from build123d import *

# Parameters (mm, degrees)
F2_R     = 0.4490128061
F3_DEPTH = 1.5875
F4_R     = 0.508


# Not quite as in the source:
# - a length typed as a fraction of an inch, garbled in the dataset ("3 / 203.2 mm" for 3/8 in), is restored


with BuildPart() as f3:
    # F2 (on Top) → F3 (new body)
    with BuildSketch(Plane.XY):
        Polygon((9.1678125, 1.27), (9.1678125, 4.0878125), (16.2321875, 4.0878125), (16.2321875, 1.27), (25.2002304245, 1.27), (25.2002304245, 17.78), (0, 17.78), (0, 1.27), align=None)
        with Locations((10.16, 7.62)):
            Circle(F2_R, mode=Mode.SUBTRACT)
        with Locations((12.7, 7.62)):
            Circle(F2_R, mode=Mode.SUBTRACT)
        with Locations((15.24, 7.62)):
            Circle(F2_R, mode=Mode.SUBTRACT)
        with Locations((5.08, 12.7)):
            Circle(F2_R, mode=Mode.SUBTRACT)
        with BuildLine():
            Line((16.4718229778, 9.1678125), (12.7, 9.1678125))
            ThreePointArc((12.7, 9.1678125), (11.9984174905, 9.4584174905), (11.7078125, 10.16))
            Line((11.7078125, 10.16), (11.7078125, 14.0486225217))
            Line((11.7078125, 14.0486225217), (13.5308885435, 15.8716985652))
            Line((13.5308885435, 15.8716985652), (18.3532987932, 11.0492883154))
            Line((18.3532987932, 11.0492883154), (16.4718229778, 9.1678125))
        make_face(mode=Mode.SUBTRACT)
        with Locations((20.32, 12.7)):
            Circle(F2_R, mode=Mode.SUBTRACT)
    extrude(amount=F3_DEPTH)

    # F4
    f4_edges = [f3.edges().sort_by_distance(p)[0] for p in [
        (25.20023, 1.27, 0.79375),
        (16.232188, 1.27, 0.79375),
        (9.167813, 1.27, 0.79375),
        (0, 1.27, 0.79375),
        (0, 17.78, 0.79375),
        (25.20023, 17.78, 0.79375),
        (11.707813, 14.048623, 0.79375),
        (13.530889, 15.871699, 0.79375),
        (18.353299, 11.049288, 0.79375),
        (16.471823, 9.167813, 0.79375),
    ]]
    fillet(f4_edges, radius=F4_R)


solid = f3.part
Build history of the part. All positions in model axes, mm. A direction names the side the tool comes from. Give positions to 0.01 mm unless a question says otherwise; leave off trailing zeros. Write each loop counter-clockwise with the first axis right and the second up, starting at its lowest first coordinate (ties: lowest second). Pieces come first, ordered by that corner, then holes. Notation, with made-up numbers: (67.25, -2) - (83.25, -2) arc R21 cw to (83.25, 6) - close; hole circle Ø7 at (-21, 84). An arc over 180 degrees is marked (long way). Use one line per item in the form item = value. Start each with the question number.
1. Probe line 1 (Y direction, x = 13.5, z = 0.55); line 2 (Y direction, x = 18, z = 0.2); line 3 (Y direction, x = 15.5, z = 0.4). List the from-to ranges inside material, lowest first. Write a range as [from, to].
2. 3-axis set-ups, long thin cutter, end or side, ignore diameter. For faces 1 (the face through (21, 1.27, 1)), 2 (the face through (11.708, 12, 1)), 3 (the face through (13, 4.088, 1)): which of +Z, -Z, +X, -X, +Y, -Y reach the whole face in a straight line?
3. Two-plate mould, pull along X, no slides. Class faces 4 (the face through (12.006, 9.451, 0.783)), 5 (the face through (5, 1.27, 1)), 6 (the face through (25.2, 9, 1)): released by +X, released by -X, zero draft, split by the parting line, or undercut.
4. Band-saw the part on B-B on y = 3.5. Write the cut outline in (x, z).
5. Drop flat-ended pins along their axis: pin 1 Ø0.5 at (x, z) = (12.5, 0.5) entering from -Y; pin 2 Ø6 at (x, y) = (21.5, 8) entering from -Z. Give the stop position or say it passes through.
6. Band-saw the part on C-C on y = 12.7. Write the cut outline in (x, z).
7. Band-saw the part on A-A on x = 10.16. Write the cut outline in (y, z).
8. Band-saw the part on D-D on z = 1.3. Count the separate pieces of the cut face and the enclosed holes in it, plus the area to 3 significant figures.
Conclusion:
q1.line_1 = [4.09, 9.17], [15.66, 17.78]
q1.line_2 = [1.27, 10.7], [11.4, 17.78]
q1.line_3 = [4.09, 7.25], [7.99, 9.17], [13.9, 17.78]
q2.face_1 = +Z, -Z, +X, -X, -Y
q2.face_2 = +Z, -Z
q2.face_3 = +Z, -Z, -Y
q3.face_4 = undercut
q3.face_5 = zero draft
q3.face_6 = released by +X
q4.outline = (0, 0) - (9.17, 0) - (9.17, 1.59) - (0, 1.59) - close; (16.23, 0) - (25.2, 0) - (25.2, 1.59) - (16.23, 1.59) - close
q5.pin_1 = 4.09
q5.pin_2 = 0
q6.outline = (0, 0) - (4.63, 0) - (4.63, 1.59) - (0, 1.59) - close; (5.53, 0) - (11.71, 0) - (11.71, 1.59) - (5.53, 1.59) - close; (16.7, 0) - (19.87, 0) - (19.87, 1.59) - (16.7, 1.59) - close; (20.77, 0) - (25.2, 0) - (25.2, 1.59) - (20.77, 1.59) - close
q7.outline = (4.09, 0) - (7.17, 0) - (7.17, 1.59) - (4.09, 1.59) - close; (8.07, 0) - (17.78, 0) - (17.78, 1.59) - (8.07, 1.59) - close
q8.separate_pieces = 1
q8.enclosed_holes = 6
q8.area = 363 mm²
